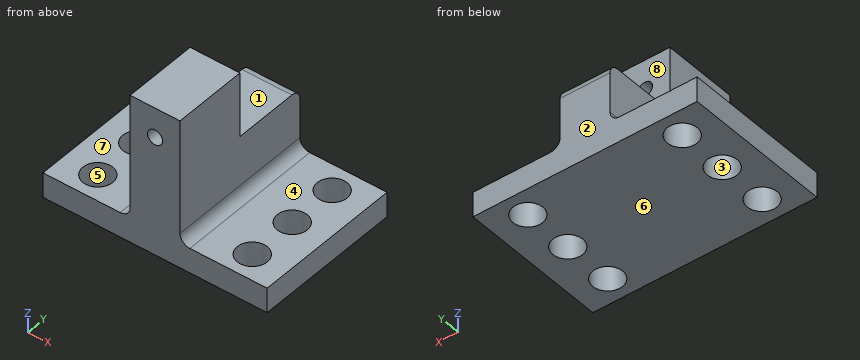
```python
from build123d import *

# Parameters (mm, degrees)
SKETCH1_W           = 45
SKETCH1_H           = 30
BASE_DEPTH          = 5
SKETCH2_W           = 10
SKETCH2_H           = 30
BOSS_EXTRUDE2_DEPTH = 25
SKETCH5_R           = 1.5
CABLE_HOLE_DEPTH    = 15
SKETCH9_R           = 3
SCREW_DEPTH         = 5
SKETCH10_W          = 15
SKETCH10_H          = 20
CUT_EXTRUDE8_DEPTH  = 10
FILLET5_R           = 2
FILLET6_R           = 2
FILLET7_R           = 2


with BuildPart() as part:
    # Sketch1 → Base (new body)
    with BuildSketch(Plane.XY):
        Rectangle(SKETCH1_W, SKETCH1_H)
    extrude(amount=BASE_DEPTH)

    # Sketch2 → Boss-Extrude2 (add)
    with BuildSketch(Plane.XY.offset(5)):
        Rectangle(SKETCH2_W, SKETCH2_H)
    extrude(amount=BOSS_EXTRUDE2_DEPTH)

    # Sketch5 → Cable hole (cut)
    with BuildSketch(Plane.XZ.offset(15)):
        with Locations((0, 24)):
            Circle(SKETCH5_R)
    extrude(amount=-CABLE_HOLE_DEPTH, mode=Mode.SUBTRACT)

    # Sketch9 → Screw (cut)
    with BuildSketch(Plane.XY.offset(5)):
        with Locations((-15.5, 10)):
            Circle(SKETCH9_R)
        with Locations((-15.5, 0)):
            Circle(SKETCH9_R)
        with Locations((-15.5, -10)):
            Circle(SKETCH9_R)
        with Locations((15.5, -10)):
            Circle(SKETCH9_R)
        with Locations((15.5, 0)):
            Circle(SKETCH9_R)
        with Locations((15.5, 10)):
            Circle(SKETCH9_R)
    extrude(amount=-SCREW_DEPTH, mode=Mode.SUBTRACT)

    # Sketch10 → Cut-Extrude8 (cut)
    with BuildSketch(Plane.ZY.offset(5)):
        with Locations((24.5, 10)):
            Rectangle(SKETCH10_W, SKETCH10_H)
    extrude(amount=-CUT_EXTRUDE8_DEPTH, mode=Mode.SUBTRACT)

    # Fillet5
    fillet5_edges = [part.edges().sort_by_distance(p)[0] for p in [
        (0, 15, 17),
    ]]
    fillet(fillet5_edges, radius=FILLET5_R)

    # Fillet6
    fillet6_edges = [part.edges().sort_by_distance(p)[0] for p in [
        (-5, 0, 5),
    ]]
    fillet(fillet6_edges, radius=FILLET6_R)

    # Fillet7
    fillet7_edges = [part.edges().sort_by_distance(p)[0] for p in [
        (5, 0, 5),
    ]]
    fillet(fillet7_edges, radius=FILLET7_R)


solid = part.part
```
Can you work these out from the model? Positions are in its coordinate system, mm. Face numbers are marked on the shaded views. A direction names the side the tool comes from. Give positions to 0.01 mm unless a question says otherwise; leave off trailing zeros. Write each loop counter-clockwise with the first axis right and the second up, starting at its lowest first coordinate (ties: lowest second). Pieces come first, ordered by that corner, then holes. Notation, with made-up numbers: (-22, -4) -> (24, -4) arc R8 ccw to (24, 2) -> close; hole circle Ø6 at (-2.75, -0.75). An arc over 180 degrees is marked (long way). Write item = value, one per line.
(1) Suppose I cut it at A-A on y = -10. Write out the boundary of the cut face in (x, z), then the cut area to 3 significant figures.
Worked out:
outline = (-22.5, 0) -> (-18.5, 0) -> (-18.5, 5) -> (-22.5, 5) -> close; (-12.5, 0) -> (12.5, 0) -> (12.5, 5) -> (7, 5) arc R2 cw to (5, 7) -> (5, 30) -> (-5, 30) -> (-5, 7) arc R2 cw to (-7, 5) -> (-12.5, 5) -> close; (18.5, 0) -> (22.5, 0) -> (22.5, 5) -> (18.5, 5) -> close; hole circle Ø3 at (0, 24)
area = 410 mm^2
(2) Suppose I cut it at C-C on x = 0. Write out the boundary of the cut face in (y, z).
Worked out:
outline = (-15, 0) -> (15, 0) -> (15, 15) arc R2 ccw to (13, 17) -> (0, 17) -> (0, 22.5) -> (-15, 22.5) -> close; (-15, 25.5) -> (0, 25.5) -> (0, 30) -> (-15, 30) -> close
(3) Thinking about a two-plate mould opening in Y: for the marked faces 1, 2 and 3, which applies, released by +Y, released by -Y, zero draft, split by the parting line, or undercut?
Worked out:
face_1 = zero draft
face_2 = released by +Y
face_3 = undercut
(4) I need wall thicknesses on probe 1 along Y at (x, z) = (15.5, 2.4); probe 2 along Z at (x, y) = (0, -3.25); probe 3 along Z at (x, y) = (19, -4). Which ranges of each line are inside material? Lowest first, please. Write a range as from..to.
Worked out:
probe_1 = -15..-13, -7..-3, 3..7, 13..15
probe_2 = 0..22.5, 25.5..30
probe_3 = 0..5
(5) For the marked faces 4, 5, 6, 7 and 8, which set-ups out of +Z, -Z, +X, -X, +Y, -Y let a thin tool reach every point of the face, with its end or its side?
Worked out:
face_4 = +Z, +X, +Y, -Y
face_5 = +Z, -Z
face_6 = -Z, +X, -X, +Y, -Y
face_7 = +Z, -X, +Y, -Y
face_8 = +Z, +X, -X, +Y
(6) I'm going to push flat-ended pins straight in: P1, Ø5, axis at x = 0, z = 24, coming from the +Y side; P2, Ø8, axis at x = 13.5, y = 1, coming from the +Z side; P3, Ø5.5, axis at x = -15.5, y = 10, coming from the -Z side; P4, Ø4, axis at y = -1, z = 14.5, coming from the +X side. Where does each tip first touch, or does it pass through?
Worked out:
P1 = 0
P2 = 5
P3 = through
P4 = 5
(7) Suppose I cut it at D-D on x = -15.5. Write out the boundary of the cut face in (y, z).
Worked out:
outline = (-15, 0) -> (-13, 0) -> (-13, 5) -> (-15, 5) -> close; (-7, 0) -> (-3, 0) -> (-3, 5) -> (-7, 5) -> close; (3, 0) -> (7, 0) -> (7, 5) -> (3, 5) -> close; (13, 0) -> (15, 0) -> (15, 5) -> (13, 5) -> close
(8) Suppose I cut it at B-B on z = 24. Write out the boundary of the cut face in (x, y).
Worked out:
outline = (-5, -15) -> (-1.5, -15) -> (-1.5, 0) -> (-5, 0) -> close; (1.5, -15) -> (5, -15) -> (5, 0) -> (1.5, 0) -> close
